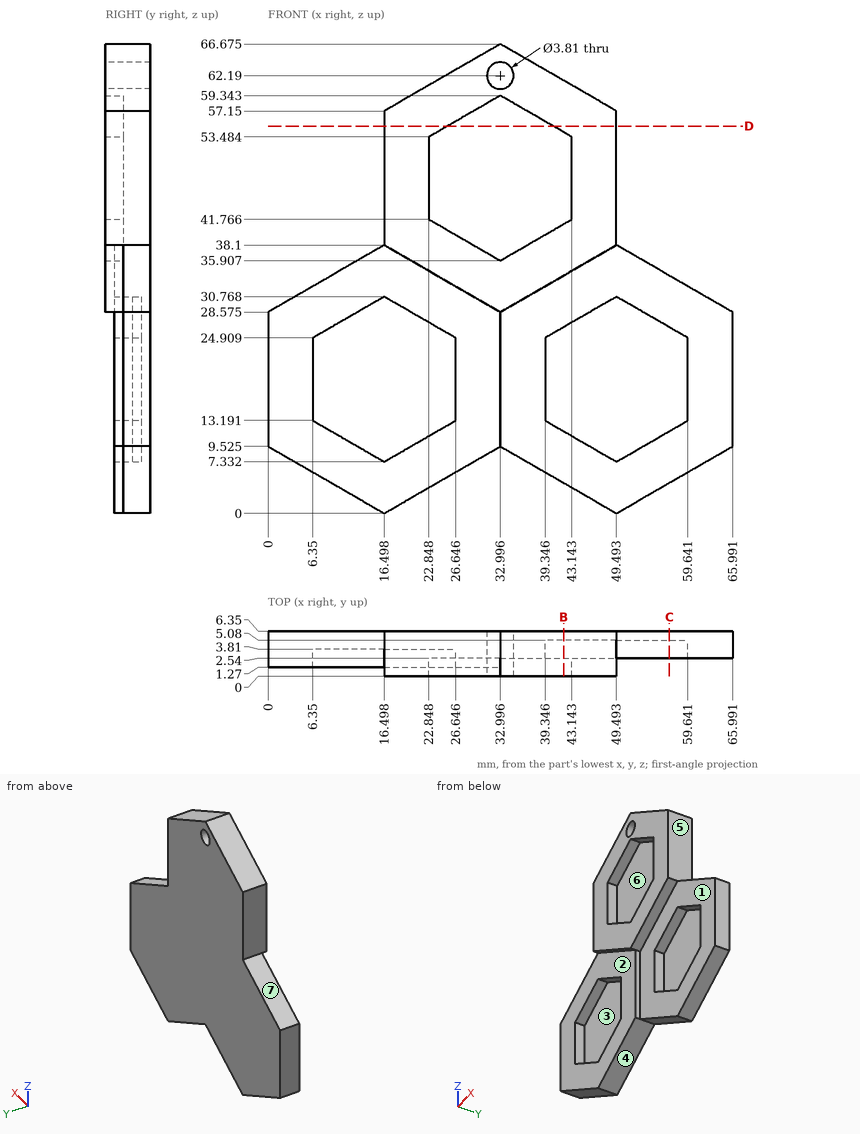
The figure shows three views and two pictorial views of one solid part (mm, origin at its lowest corner). Answer the questions. A direction names the side the tool comes from. Coordinates: 2 decimals unless noted, no trailing zeros. Loops run counter-clockwise (first coordinate to the right, second up) from the corner with the lowest first, then second, coordinate; pieces in that order, holes last. Notation, with made-up numbers: (62, 7.25) -> (70, 7.25) arc R17 cw to (70, 28.25) -> close; hole circle Ø8 at (-39, 11.5). An arc over 180 degrees is marked (long way). Return JSON: item names as keys, results as strings. Group by question number.
(1) Find the intervals of material crossed by probe 1 along X at (y, z) = (1.75, 53); probe 2 along Y at (x, z) = (57.5, 9.5); probe 3 along Y at (x, z) = (47, 15), in increasing order. Write a range as from..to.
(2) Which of the six approach directions +Z, -Z, +X, -X, +Y, -Y give full straight-line access (tool end or side, diameter ignored) to the marked faces 1, 2 and 3?
(3) A cutting plane is placed at D-D on z = 55. Write down the section's boundary in (x, y), and give its area (3 significant figures).
(4) Given pin 1 Ø1.3 at (y, z) = (1, 45.5) entering from -X; pin 2 Ø3 at (y, z) = (3.5, 35.5) entering from -X (1 decimal); pin 3 Ø10 at (x, z) = (55.5, 28) entering from -Y, each flat-ended and moving along its own axis, determine where each tip first touches the part or whether it passes through.
(5) A cutting plane is placed at C-C on x = 57. Write down the section's boundary in (y, z).
(6) Determine the mould class of the marked faces 4, 5, 6 and 7 for opening direction Z: released by +Z, released by -Z, zero draft, split by the parting line, or undercut.
(7) A cutting plane is placed at B-B on x = 42. Write down the section's boundary in (y, z).
The answers:
{
 "1": {"probe 1": "x = 16.5..22.85, 43.14..49.49", "probe 2": "y = 2.54..6.35", "probe 3": "y = 5.08..6.35"},
 "2": {"face 1": "-Z, +X, -Y", "face 2": "-Z, -X, -Y", "face 3": "-Y"},
 "3": {"outline": "(16.5, 0) -> (25.47, 0) -> (25.47, 2.54) -> (40.52, 2.54) -> (40.52, 0) -> (49.49, 0) -> (49.49, 6.35) -> (16.5, 6.35) -> close", "area": "171 mm^2"},
 "4": {"pin 1": "stops at x = 16.5", "pin 2": "stops at x = 9.4", "pin 3": "stops at y = 2.54"},
 "5": {"outline": "(2.54, 4.33) -> (6.35, 4.33) -> (6.35, 33.77) -> (2.54, 33.77) -> (2.54, 26.43) -> (5.08, 26.43) -> (5.08, 11.67) -> (2.54, 11.67) -> close"},
 "6": {"face 4": "released by -Z", "face 5": "zero draft", "face 6": "undercut", "face 7": "released by +Z"},
 "7": {"outline": "(0, 33.77) -> (2.54, 33.77) -> (2.54, 26.44) -> (5.08, 26.44) -> (5.08, 11.66) -> (2.54, 11.66) -> (2.54, 4.33) -> (6.35, 4.33) -> (6.35, 61.48) -> (0, 61.48) -> (0, 54.14) -> (2.54, 54.14) -> (2.54, 41.11) -> (0, 41.11) -> close"}
}
